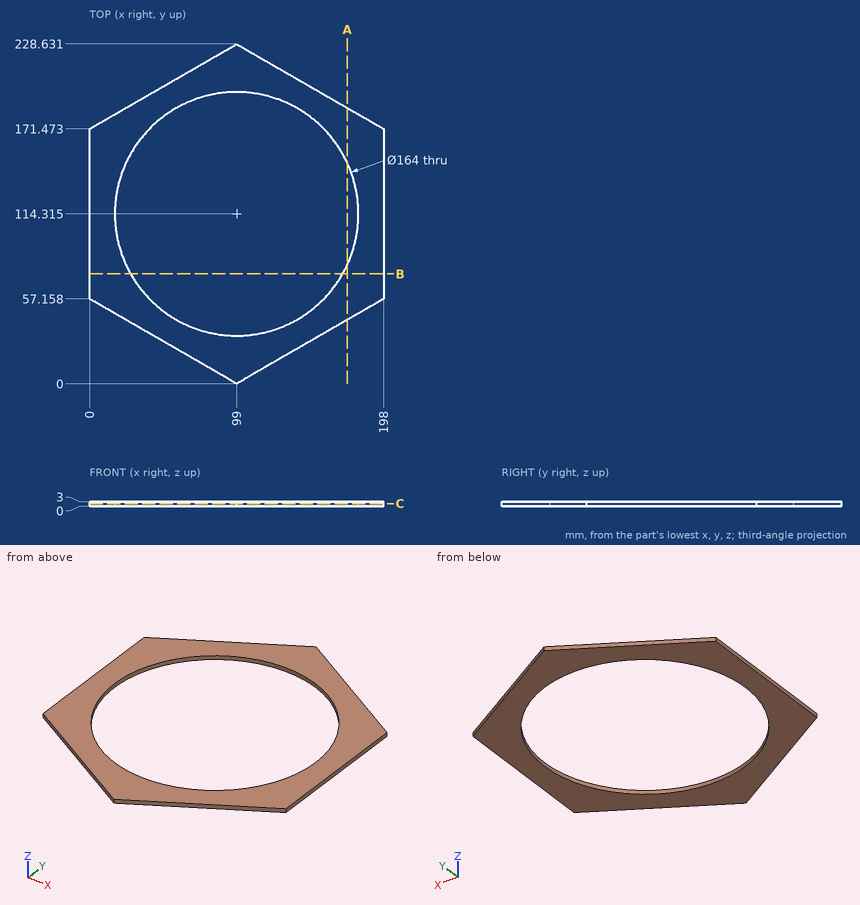
Geometry check sheet. Reference: drawing and pictorial views, mm from the part's lowest x, y, z. Coordinates: 2 decimals unless noted, no trailing zeros. Order: outer loops, then holes, each group sorted by start corner. A loop starts at its lowest first (then second) coordinate and runs counter-clockwise, first axis right, second up. Notation, with made-up numbers: (38.5, 89.5) -> (52.5, 89.5) arc R12 ccw to (52.5, 93.5) -> close; hole circle Ø4 at (-8.5, 23.25). An arc over 180 degrees is marked (long way). Put each result on its own line as item: value. Start each with the question number.
1) Cross-section at B-B (y = 74). Enter the section's corners in (x, z) (1 decimal).
2) Material ranges on L1, parallel to Y at x = 42.5, z = 2.1 (1 decimal); L2, parallel to X at y = 90, z = 2.35; L3, parallel to X at y = 182, z = 0.25 (1 decimal), recorded low to high.
3) Go/stop test with a flat-tipped pin: pin 1 (1 mm diameter, centred on x = 32, z = 0.5, fed in from -Y). Record where the tip stops, or that it passes through.
4) Cross-section at C-C (z = 1.7). Enter the section's corners in (x, y) (1 decimal).
5) Cross-section at A-A (x = 173.5). Enter the section's corners in (y, z) (1 decimal), plus the area to 3 significant figures.
Geometry check:
1. outline: (0, 0) -> (27.6, 0) -> (27.6, 3) -> (0, 3) -> close; (170.4, 0) -> (198, 0) -> (198, 3) -> (170.4, 3) -> close
2. L1: y = 32.6 to 54.9, 173.7 to 196
2. L2: x = 0 to 20.69, 177.31 to 198
2. L3: x = 18.2 to 52.7, 145.3 to 179.8
3. pin 1: stops at y = 38.39
4. outline: (0, 57.2) -> (99, 0) -> (198, 57.2) -> (198, 171.5) -> (99, 228.6) -> (0, 171.5) -> close; hole circle Ø164 at (99, 114.3)
5. outline: (43, 0) -> (80.1, 0) -> (80.1, 3) -> (43, 3) -> close; (148.6, 0) -> (185.6, 0) -> (185.6, 3) -> (148.6, 3) -> close
5. area: 222 mm^2
